from build123d import *

# Parameters (mm, degrees)
SKETCH1_W                                     = 50
SKETCH1_H                                     = 60
BOSS_EXTRUDE1_DEPTH                           = 10
FILLET1_R                                     = 5
CUT_EXTRUDE1_DEPTH                            = 10
CSK_FOR_M5_COUNTERSUNK_FLAT_HEAD1_D           = 5.5
CSK_FOR_M5_COUNTERSUNK_FLAT_HEAD1_DEPTH       = 30
CSK_FOR_M5_COUNTERSUNK_FLAT_HEAD1_CSINK_D     = 10.4
CSK_FOR_M5_COUNTERSUNK_FLAT_HEAD1_CSINK_ANGLE = 90
CSK_FOR_M5_COUNTERSUNK_FLAT_HEAD1_TIP         = 1.652366702


with BuildPart() as part:
    # Sketch1 → Boss-Extrude1 (new body)
    with BuildSketch(Plane.XY):
        with Locations((25, 30)):
            Rectangle(SKETCH1_W, SKETCH1_H)
    extrude(amount=BOSS_EXTRUDE1_DEPTH)

    # Fillet1
    fillet1_edges = [part.edges().sort_by_distance(p)[0] for p in [
        (0, 60, 5),
        (50, 60, 5),
        (50, 0, 5),
        (0, 0, 5),
    ]]
    fillet(fillet1_edges, radius=FILLET1_R)

    # Sketch2 → Cut-Extrude1 (cut)
    with BuildSketch(Plane.XY.offset(10)):
        with BuildLine():
            Line((12.5, 20), (12.5, 8))
            ThreePointArc((12.5, 8), (8.75, 4.25), (5, 8))
            Line((5, 8), (5, 20))
            ThreePointArc((5, 20), (8.75, 23.75), (12.5, 20))
        make_face()
        with BuildLine():
            Line((37.5, 40), (37.5, 52))
            ThreePointArc((37.5, 52), (41.25, 55.75), (45, 52))
            Line((45, 52), (45, 40))
            ThreePointArc((45, 40), (41.25, 36.25), (37.5, 40))
        make_face()
        with BuildLine():
            Line((37.5, 20), (37.5, 8))
            ThreePointArc((37.5, 8), (41.25, 4.25), (45, 8))
            Line((45, 8), (45, 20))
            ThreePointArc((45, 20), (41.25, 23.75), (37.5, 20))
        make_face()
        with BuildLine():
            Line((12.5, 40), (12.5, 52))
            ThreePointArc((12.5, 52), (8.75, 55.75), (5, 52))
            Line((5, 52), (5, 40))
            ThreePointArc((5, 40), (8.75, 36.25), (12.5, 40))
        make_face()
    extrude(amount=-CUT_EXTRUDE1_DEPTH, mode=Mode.SUBTRACT)

    # CSK for M5 Countersunk Flat Head1
    with Locations(Plane.XY.offset(10)):
        with Locations((25, 38), (25, 22)):
            CounterSinkHole(CSK_FOR_M5_COUNTERSUNK_FLAT_HEAD1_D / 2, CSK_FOR_M5_COUNTERSUNK_FLAT_HEAD1_CSINK_D / 2, depth=CSK_FOR_M5_COUNTERSUNK_FLAT_HEAD1_DEPTH, counter_sink_angle=CSK_FOR_M5_COUNTERSUNK_FLAT_HEAD1_CSINK_ANGLE)
            with Locations((0, 0, -(CSK_FOR_M5_COUNTERSUNK_FLAT_HEAD1_DEPTH + CSK_FOR_M5_COUNTERSUNK_FLAT_HEAD1_TIP / 2))):  # 118° drill point
                Cone(0, CSK_FOR_M5_COUNTERSUNK_FLAT_HEAD1_D / 2, CSK_FOR_M5_COUNTERSUNK_FLAT_HEAD1_TIP, mode=Mode.SUBTRACT)


solid = part.part
Verification items for the finished model (mm, model axes). A direction names the side the tool comes from. Coordinates: 2 decimals unless noted, no trailing zeros. Order: outer loops, then holes, each group sorted by start corner. A loop starts at its lowest first (then second) coordinate and runs counter-clockwise, first axis right, second up. Notation, with made-up numbers: (44, 37.25) -> (53, 37.25) arc R19 ccw to (53, 44.25) -> close; hole circle Ø2 at (-10.75, 39.25). An arc over 180 degrees is marked (long way). Use CSV: the item, a comma, the result in double quotes. Start each with the question number.
Q1. Section check D-D, the plane z = 9. Record the cut outline in (x, y).
Q2. Section check B-B, the plane z = 2.5. Record the cut outline in (x, y), and give its area (3 significant figures).
Q3. Draft check along X on faces 1 (the cylindrical face through (27.027, 39.859, 3.722)), 2 (the flat face through (25, 30, 10)), 3 (the cylindrical face through (48, 1, 5)). Enter one of: +X half, -X half, draft (parallel to the pull), parting line (faces both ways), or undercut.
Q4. Section check A-A, the plane y = 45. Record the cut outline in (x, z).
Q5. Depth check by flat-ended pin: P1, Ø6.5, axis at x = 25, y = 22, coming from the +Z side. Enter the tip coordinate at first touch or a pass-through.
Q6. Section check C-C, the plane x = 8.75. Record the cut outline in (y, z).
Q7. Thickness scan on line 1 along Y through (x, z) = (25, 4); line 2 along X through (y, z) = (13, 3); line 3 along Y through (x, z) = (8.5, 8.25). Record the ranges inside material, lowest first.
Q8. Tool access check on faces 4 (the flat face through (5, 14, 5)), 5 (the conical face through (23.46, 40.42, 7.67)). Record the directions out of +Z, -Z, +X, -X, +Y, -Y that give a thin tool (end or side, any length) a straight path to the whole face; none if there is none.
Returned:
1,outline,"(0, 5) arc R5 ccw to (5, 0) -> (45, 0) arc R5 ccw to (50, 5) -> (50, 55) arc R5 ccw to (45, 60) -> (5, 60) arc R5 ccw to (0, 55) -> close; hole (5, 8) arc R3.75 ccw to (12.5, 8) -> (12.5, 20) arc R3.75 ccw to (5, 20) -> close; hole (5, 40) arc R3.75 ccw to (12.5, 40) -> (12.5, 52) arc R3.75 ccw to (5, 52) -> close; hole circle Ø8.4 at (25, 22); hole circle Ø8.4 at (25, 38); hole (37.5, 8) arc R3.75 ccw to (45, 8) -> (45, 20) arc R3.75 ccw to (37.5, 20) -> close; hole (37.5, 40) arc R3.75 ccw to (45, 40) -> (45, 52) arc R3.75 ccw to (37.5, 52) -> close"
2,outline,"(0, 5) arc R5 ccw to (5, 0) -> (45, 0) arc R5 ccw to (50, 5) -> (50, 55) arc R5 ccw to (45, 60) -> (5, 60) arc R5 ccw to (0, 55) -> close; hole (5, 8) arc R3.75 ccw to (12.5, 8) -> (12.5, 20) arc R3.75 ccw to (5, 20) -> close; hole (5, 40) arc R3.75 ccw to (12.5, 40) -> (12.5, 52) arc R3.75 ccw to (5, 52) -> close; hole circle Ø5.5 at (25, 22); hole circle Ø5.5 at (25, 38); hole (37.5, 8) arc R3.75 ccw to (45, 8) -> (45, 20) arc R3.75 ccw to (37.5, 20) -> close; hole (37.5, 40) arc R3.75 ccw to (45, 40) -> (45, 52) arc R3.75 ccw to (37.5, 52) -> close"
2,area,"2,390 mm^2"
3,face 1,"undercut"
3,face 2,"draft"
3,face 3,"+X half"
4,outline,"(0, 0) -> (5, 0) -> (5, 10) -> (0, 10) -> close; (12.5, 0) -> (37.5, 0) -> (37.5, 10) -> (12.5, 10) -> close; (45, 0) -> (50, 0) -> (50, 10) -> (45, 10) -> close"
5,P1,"stops at z = 8.05"
6,outline,"(0, 0) -> (4.25, 0) -> (4.25, 10) -> (0, 10) -> close; (23.75, 0) -> (36.25, 0) -> (36.25, 10) -> (23.75, 10) -> close; (55.75, 0) -> (60, 0) -> (60, 10) -> (55.75, 10) -> close"
7,line 1,"y = 0 to 19.25, 24.75 to 35.25, 40.75 to 60"
7,line 2,"x = 0 to 5, 12.5 to 37.5, 45 to 50"
7,line 3,"y = 0 to 4.26, 23.74 to 36.26, 55.74 to 60"
8,face 4,"+Z, -Z"
8,face 5,"+Z"
